Check sheet for the modelled part. Datum: model origin and axes. Units: mm. A direction names the side the tool comes from. Round coordinates to 2 decimals unless told otherwise and drop trailing zeros. Order: outer loops, then holes, each group sorted by start corner. A loop starts at its lowest first (then second) coordinate and runs counter-clockwise, first axis right, second up.
(1) Thickness scan on probe 1 along X at (y, z) = (-8, 12.7); probe 2 along Z at (x, y) = (25.4, -10.75); probe 3 along X at (y, z) = (11, 8). Record the ranges inside material, lowest first.
(2) Tool access check on faces 4 (the flat face through (12.7, 0, 4)), 5 (the flat face through (25.4, 0, 13)), 6 (the flat face through (25, 12.7, 18)), 7 (the flat face through (23, 6.35, 13)), 8 (the flat face through (19, 0, 19.05)). Record the directions out of +Z, -Z, +X, -X, +Y, -Y that give a thin tool (end or side, any length) a straight path to the whole face; none if there is none.
(3) Sectioned sample at C-C, the plane y = -11. Enter the section's corners in (x, z).
(4) Sectioned sample at A-A, the plane y = -2.75. Enter the section's corners in (x, z).
(5) Mould release check, pull along X, two halves, no side actions. Record for faces 1 (the flat face through (19, 0, 6.35)), 2 (the flat face through (0, 0, 13)), 3 (the flat face through (23, -6.35, 13)): released by +X, released by -X, zero draft, split by the parting line, or undercut.
(6) Sectioned sample at B-B, the plane z = 12.7. Enter the section's corners in (x, y), and give its area (3 significant figures).
(7) Sectioned sample at D-D, the plane x = 5.5. Enter the section's corners in (y, z), and give its area (3 significant figures).
(8) Depth check by flat-ended pin: pin 1 (5.5 mm diameter, centred on x = 23, z = 15, fed in from +Y); pin 2 (12 mm diameter, centred on x = 21, y = 4, fed in from +Z); pin 3 (6 mm diameter, centred on x = 25.4, z = 12.7, fed in from +Y); pin 4 (2 mm diameter, centred on x = 23.5, z = 3.5, fed in from +Y). Enter the tip coordinate at first touch or a pass-through.
```python
from build123d import *

# Parameters (mm, degrees)
F1_DEPTH      = 12.7
F0_W          = 6.35
F0_H          = 12.7
F2_DEPTH      = 25.4
F3_R          = 6.35
F3_R_2        = 5.08
F4_DEPTH      = 6.35
F4_DEPTH_BACK = 19.05


with BuildPart() as f1:
    # F0 (on Right) → F1 (new body)
    with BuildSketch(Plane.YZ):
        Polygon((-6.35, 19.05), (0, 19.05), (0, 25.4), (-6.35, 25.4), (-12.7, 19.05), (-12.7, 0), (0, 0), (0, 6.35), (-6.35, 6.35), align=None)
        Polygon((0, 25.4), (0, 19.05), (6.35, 19.05), (6.35, 6.35), (0, 6.35), (0, 0), (12.7, 0), (12.7, 19.05), (6.35, 25.4), align=None)
    extrude(amount=F1_DEPTH)

    # F0 (on Right) → F2 (join)
    with BuildSketch(Plane.YZ):
        with Locations((3.175, 12.7)):
            Rectangle(F0_W, F0_H)
        with Locations((-3.175, 12.7)):
            Rectangle(F0_W, F0_H)
    extrude(amount=F2_DEPTH)

    # F3 (on face) → F4 (join, two sides)
    with BuildSketch(Plane.XZ.offset(6.35)) as f4_sk:
        with Locations((25.4, 12.7)):
            Circle(F3_R)
        with Locations((25.4, 12.7)):
            Circle(F3_R_2, mode=Mode.SUBTRACT)
    extrude(amount=F4_DEPTH)
    extrude(f4_sk.sketch, amount=-F4_DEPTH_BACK)


solid = f1.part
```
Derived:
1. probe 1: x = 0 to 12.7, 19.05 to 20.32, 30.48 to 31.75
1. probe 2: z = 6.35 to 7.62, 17.78 to 19.05
1. probe 3: x = 0 to 12.7, 21.13 to 23.47, 27.33 to 29.67
2. face 4: none
2. face 5: +Y, -Y
2. face 6: +Z, -Z, +X, -X, +Y
2. face 7: +Y
2. face 8: +Z, +X, +Y, -Y
3. outline: (0, 0) - (12.7, 0) - (12.7, 20.75) - (0, 20.75) - close; circle Ø12.7 at (25.4, 12.7); hole circle Ø10.16 at (25.4, 12.7)
4. outline: (0, 0) - (12.7, 0) - (12.7, 6.35) - (25.4, 6.35) arc R6.35 ccw to (25.4, 19.05) - (12.7, 19.05) - (12.7, 25.4) - (0, 25.4) - close; hole (25.4, 7.62) arc R5.08 ccw to (25.4, 17.78) - close
5. face 1: zero draft
5. face 2: released by -X
5. face 3: undercut
6. outline: (0, -12.7) - (12.7, -12.7) - (12.7, -6.35) - (19.05, -6.35) - (19.05, -12.7) - (20.32, -12.7) - (20.32, -6.35) - (25.4, -6.35) - (25.4, 6.35) - (20.32, 6.35) - (20.32, 12.7) - (19.05, 12.7) - (19.05, 6.35) - (12.7, 6.35) - (12.7, 12.7) - (0, 12.7) - close; (30.48, -12.7) - (31.75, -12.7) - (31.75, 12.7) - (30.48, 12.7) - close
6. area: 532 mm2
7. outline: (-12.7, 0) - (12.7, 0) - (12.7, 19.05) - (6.35, 25.4) - (-6.35, 25.4) - (-12.7, 19.05) - close
7. area: 605 mm2
8. pin 1: stops at y = 12.7
8. pin 2: stops at z = 19.05
8. pin 3: stops at y = 6.35
8. pin 4: passes through
